Geometry check sheet. Reference: the model listing, model coordinates, mm. A direction names the side the tool comes from. Give positions to 0.01 mm unless a question says otherwise; leave off trailing zeros. Loops run counter-clockwise (first coordinate to the right, second up) from the corner with the lowest first, then second, coordinate; pieces in that order, holes last. Notation, with made-up numbers: (38.25, 37) -> (85.25, 37) arc R20 ccw to (85.25, 43) -> close; hole circle Ø2 at (63.5, 24.5). An arc over 180 degrees is marked (long way). Write item = value, one per line.
```python
from build123d import *

# Parameters (mm, degrees)
SKETCH2_W           = 40
SKETCH2_H           = 15
BOSS_EXTRUDE2_DEPTH = 5
CHAMFER1_SIZE       = 3
SKETCH5_R           = 7
SKETCH5_R_2         = 6
BOSS_EXTRUDE4_DEPTH = 4


with BuildPart() as part:
    # Sketch2 → Boss-Extrude2 (new body)
    with BuildSketch(Plane(origin=(0, 4, 0), x_dir=(1, 0, 0), z_dir=(0, 1, 0))):
        Rectangle(SKETCH2_W, SKETCH2_H)
    extrude(amount=BOSS_EXTRUDE2_DEPTH)

    # Chamfer1
    chamfer1_edges = [part.edges().sort_by_distance(p)[0] for p in [
        (-20, 9, 0),
        (0, 9, 7.5),
        (20, 9, 0),
        (0, 9, -7.5),
    ]]
    chamfer(chamfer1_edges, length=CHAMFER1_SIZE)

    # Sketch5 → Boss-Extrude4 (add)
    with BuildSketch(Plane(origin=(0, 4, 0), x_dir=(-1, 0, 0), z_dir=(0, -1, 0))):
        with Locations(Location((0, 0, 0), (0, 0, 270))):
            Circle(SKETCH5_R)
        with Locations(Location((0, 0, 0), (0, 0, 90))):
            Circle(SKETCH5_R_2, mode=Mode.SUBTRACT)
    extrude(amount=BOSS_EXTRUDE4_DEPTH)


solid = part.part
```
Item 1: Section check D-D, the plane z = -6.5. Record the cut outline in (x, y), plus the area to 3 significant figures.
Answer:
outline = (-20, 4) -> (-2.6, 4) -> (-2.6, 0) -> (2.6, 0) -> (2.6, 4) -> (20, 4) -> (20, 6) -> (19, 7) -> (-19, 7) -> (-20, 6) -> close
area = 140 mm^2
Item 2: Gauge pin test, flat ends, axial feed: pin 1 (5 mm diameter, centred on x = -0.5, y = 1, fed in from +Z); pin 2 (1.5 mm diameter, centred on x = -4, y = 7, fed in from +Z); pin 3 (1 mm diameter, centred on x = -8, z = -5.5, fed in from +Y). Record the tip position at first contact, or that the pin passes through.
Answer:
pin_1 = 7
pin_2 = 7.25
pin_3 = 8.5
Item 3: Draft check along Z on faces 3 (the flat face through (-18, 8, 0)), 4 (the cylindrical face through (1.802, 2.028, -5.723)), 5 (the flat face through (-0.3, 7.5, 6)). Enter one of: +Z half, -Z half, draft (parallel to the pull), parting line (faces both ways), or undercut.
Answer:
face_3 = draft
face_4 = undercut
face_5 = +Z half
Item 4: Thickness scan on L1, parallel to X at y = 2.6, z = 0; L2, parallel to Y at x = -10.5, z = 3; L3, parallel to X at y = 0.75, z = 1.75. Record the ranges inside material, lowest first. Write a range as [from, to].
Answer:
L1 = [-7, -6], [6, 7]
L2 = [4, 9]
L3 = [-6.78, -5.74], [5.74, 6.78]
Item 5: Section check C-C, the plane y = 2.75. Record the cut outline in (x, z).
Answer:
outline = circle Ø14 at (0, 0); hole circle Ø12 at (0, 0)
Item 6: Section check B-B, the plane x = 0. Record the cut outline in (y, z), plus the area to 3 significant figures.
Answer:
outline = (0, -7) -> (4, -7) -> (4, -7.5) -> (6, -7.5) -> (9, -4.5) -> (9, 4.5) -> (6, 7.5) -> (4, 7.5) -> (4, 7) -> (0, 7) -> (0, 6) -> (4, 6) -> (4, -6) -> (0, -6) -> close
area = 74.0 mm^2
Item 7: Section check A-A, the plane z = 0. Record the cut outline in (x, y).
Answer:
outline = (-20, 4) -> (-7, 4) -> (-7, 0) -> (-6, 0) -> (-6, 4) -> (6, 4) -> (6, 0) -> (7, 0) -> (7, 4) -> (20, 4) -> (20, 6) -> (17, 9) -> (-17, 9) -> (-20, 6) -> close
Item 8: Tool access check on faces 1 (the flat face through (-20, 5, 0)), 2 (the flat face through (0, 4, 0)). Record the directions out of +Z, -Z, +X, -X, +Y, -Y that give a thin tool (end or side, any length) a straight path to the whole face; none if there is none.
Answer:
face_1 = +Z, -Z, -X, +Y, -Y
face_2 = -Y
